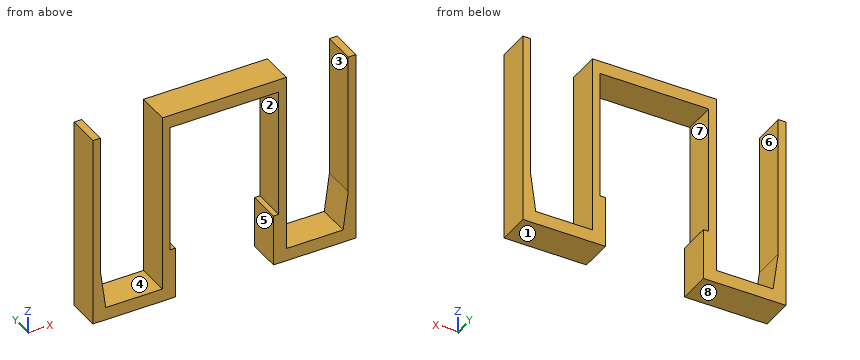
```python
from build123d import *

# Parameters (mm, degrees)
BOSS_EXTRUDE1_DEPTH = 12.7


with BuildPart() as part:
    # Sketch1 → Boss-Extrude1 (new, symmetric)
    with BuildSketch(Plane(origin=(0, 0, 0), x_dir=(1, 0, 0), z_dir=(0, 1, 0))):
        Polygon((-92.1, 130), (-96.1, 100), (-96.1, -10), (-102.1, -10), (-102.1, 140), (-38.1, 140), (-38.1, 100), (-42.1, 100), (-42.1, 0), (42.1, 0), (42.1, 100), (38.1, 100), (38.1, 140), (102.1, 140), (102.1, -10), (96.1, -10), (96.1, 100), (92.1, 130), (48.1, 130), (48.1, -10), (-48.1, -10), (-48.1, 130), align=None)
    extrude(amount=BOSS_EXTRUDE1_DEPTH, both=True)


solid = part.part
```
Model file for the job. Use its own axes, mm. Face numbers are marked on the shaded views. A direction names the side the tool comes from. Give positions to 0.01 mm unless a question says otherwise; leave off trailing zeros. Write each loop counter-clockwise with the first axis right and the second up, starting at its lowest first coordinate (ties: lowest second). Pieces come first, ordered by that corner, then holes. Notation, with made-up numbers: M 57.5,56.25 L 109.5,56.25 A13 cw 109.5,75.25 Z; hole C 3.5,80 d2. An arc over 180 degrees is marked long. Use a Markdown table: item, result.
1) Cut at D-D (x = 16). List the corners of the cut face in (y, z), and give its area (3 significant figures).
Responses:
| item | result |
|---|---|
| outline | M -12.7,0 L 12.7,0 L 12.7,10 L -12.7,10 Z |
| area | 254 mm2 |
2) Cut at A-A (z = -34). List the corners of the cut face in (x, y), and give its area (3 significant figures).
Responses:
| item | result |
|---|---|
| outline | M -102.1,-12.7 L -96.1,-12.7 L -96.1,12.7 L -102.1,12.7 Z; M -48.1,-12.7 L -42.1,-12.7 L -42.1,12.7 L -48.1,12.7 Z; M 42.1,-12.7 L 48.1,-12.7 L 48.1,12.7 L 42.1,12.7 Z; M 96.1,-12.7 L 102.1,-12.7 L 102.1,12.7 L 96.1,12.7 Z |
| area | 610 mm2 |
3) Drill centre lines: line 1 (X direction, y = -3.5, z = -77); line 2 (X direction, y = -11.5, z = -114); line 3 (Z direction, x = -34, y = 11.75). Where is each one in solid material? Low to high. Write a range as from..to.
Responses:
| item | result |
|---|---|
| line 1 | x = -102.1..-96.1, -48.1..-42.1, 42.1..48.1, 96.1..102.1 |
| line 2 | x = -102.1..-94.23, -48.1..-38.1, 38.1..48.1, 94.23..102.1 |
| line 3 | z = 0..10 |
4) Tool access for the marked faces 5, 6, 7 and 8: list every direction of +Z, -Z, +X, -X, +Y, -Y with a clear straight run to the whole face (end or side of a thin tool).
Responses:
| item | result |
|---|---|
| face 5 | -Z, +Y, -Y |
| face 6 | +Z, +Y, -Y |
| face 7 | +Y, -Y |
| face 8 | -Z, +X, -X, +Y, -Y |
5) Cut at C-C (z = -117.5). List the corners of the cut face in (x, y).
Responses:
| item | result |
|---|---|
| outline | M -102.1,-12.7 L -93.77,-12.7 L -93.77,12.7 L -102.1,12.7 Z; M -48.1,-12.7 L -38.1,-12.7 L -38.1,12.7 L -48.1,12.7 Z; M 38.1,-12.7 L 48.1,-12.7 L 48.1,12.7 L 38.1,12.7 Z; M 93.77,-12.7 L 102.1,-12.7 L 102.1,12.7 L 93.77,12.7 Z |
6) Cut at B-B (y = 8.25). List the corners of the cut face in (x, z).
Responses:
| item | result |
|---|---|
| outline | M -102.1,-140 L -38.1,-140 L -38.1,-100 L -42.1,-100 L -42.1,0 L 42.1,0 L 42.1,-100 L 38.1,-100 L 38.1,-140 L 102.1,-140 L 102.1,10 L 96.1,10 L 96.1,-100 L 92.1,-130 L 48.1,-130 L 48.1,10 L -48.1,10 L -48.1,-130 L -92.1,-130 L -96.1,-100 L -96.1,10 L -102.1,10 Z |
7) Pull direction Z, two halves, no side cores. Call the marked faces 1, 2, 3 and 4: +Z half, -Z half, draft (parallel to the pull), parting line (faces both ways), or undercut.
Responses:
| item | result |
|---|---|
| face 1 | -Z half |
| face 2 | undercut |
| face 3 | draft |
| face 4 | +Z half |
8) Pin check, flat tips, straight feed: pin 1 (12.5 mm diameter, centred on x = -75, y = 5.5, fed in from +Z); pin 2 (6 mm diameter, centred on x = -13, y = 3.5, fed in from -Z). Stop position of each tip, or through.
Responses:
| item | result |
|---|---|
| pin 1 | stops at z = -130 |
| pin 2 | stops at z = 0 |
